For this review, take the finished solid that the model builds, in its own axes (mm). A direction names the side the tool comes from. Coordinates: 2 decimals unless noted, no trailing zeros. Order: outer loops, then holes, each group sorted by start corner. A loop starts at its lowest first (then second) coordinate and runs counter-clockwise, first axis right, second up. Notation, with made-up numbers: (55.25, -32) -> (60.25, -32) arc R36 ccw to (60.25, 4) -> close; hole circle Ø9 at (88.5, 14). An arc over 180 degrees is marked (long way). Answer as a JSON object with one key per item and string values. Group by question number.
1) For pin 1 (2 mm diameter, centred on x = -1, y = 9.5, fed in from +Z); pin 2 (2 mm diameter, centred on x = -1, y = 10.5, fed in from -Z), all flat-tipped, find the tip position at first contact; note any pin that passes through.
2) Add section B-B, the plane x = -4.5. Write out the cut boundary in (y, z), then the cut area to 3 significant figures.
3) Wall thickness on L1, parallel to Z at x = -3, y = 8; L2, parallel to X at y = 12, z = -0.25; L3, parallel to X at y = 10.5, z = -1: over which ranges is each line inside the solid? List them lowest first.
4) Add section A-A, the plane z = -2.75. Write out the cut boundary in (x, y).
5) Machinability: for faces 1 (the flat face through (-4, 15.5, -4.7)), 2 (the cylindrical face through (-6, 8, 0)), 3 (the flat face through (0, 8, -4.95)), which of the approach directions +Z, -Z, +X, -X, +Y, -Y give a long, thin tool a straight path to every point of the face, cutting with its end or side? Answer none if there is none.
6) Add section C-C, the plane y = 9.25. Write out the cut boundary in (x, z), then the cut area to 3 significant figures.
from build123d import *

# Parameters (mm, degrees)
BOSS_EXTRUDE1_DEPTH = 15.5
SKETCH2_W           = 12
SKETCH2_H           = 10
BOSS_EXTRUDE2_DEPTH = 9


with BuildPart() as part:
    # Sketch1 → Boss-Extrude1 (new body)
    with BuildSketch(Plane(origin=(0, 0, 0), x_dir=(1, 0, 0), z_dir=(0, 1, 0))):
        with BuildLine():
            Line((-3.390796367, 4.95), (3.390796367, 4.95))
            ThreePointArc((3.390796367, 4.95), (6, 0), (3.390796367, -4.95))
            Line((3.390796367, -4.95), (-3.390796367, -4.95))
            ThreePointArc((-3.390796367, -4.95), (-6, 0), (-3.390796367, 4.95))
        make_face()
    extrude(amount=BOSS_EXTRUDE1_DEPTH)

    # Sketch2 → Boss-Extrude2 (add)
    with BuildSketch(Plane(origin=(0, 15.5, 0), x_dir=(1, 0, 0), z_dir=(0, 1, 0))):
        Rectangle(SKETCH2_W, SKETCH2_H)
    extrude(amount=BOSS_EXTRUDE2_DEPTH)


solid = part.part
Output values:
{
 "1": {"pin 1": "stops at z = 4.95", "pin 2": "stops at z = -4.95"},
 "2": {"outline": "(0, -3.97) -> (15.5, -3.97) -> (15.5, -5) -> (24.5, -5) -> (24.5, 5) -> (15.5, 5) -> (15.5, 3.97) -> (0, 3.97) -> close", "area": "213 mm²"},
 "3": {"L1": "z = -4.95 to 4.95", "L2": "x = -5.99 to 5.99", "L3": "x = -5.92 to 5.92"},
 "4": {"outline": "(-6, 15.5) -> (-5.33, 15.5) -> (-5.33, 0) -> (5.33, 0) -> (5.33, 15.5) -> (6, 15.5) -> (6, 24.5) -> (-6, 24.5) -> close"},
 "5": {"face 1": "-Z, -Y", "face 2": "-X, -Y", "face 3": "-Z, +X, -X, -Y"},
 "6": {"outline": "(-3.39, -4.95) -> (3.39, -4.95) arc R6 ccw to (3.39, 4.95) -> (-3.39, 4.95) arc R6 ccw to start", "area": "103 mm²"}
}
